Autodesk Inventor part; units mm, degrees
ref_plane "XZ Plane" through (0, 0, 0) normal (0, 1, 0) x (-1, 0, 0)
ref_plane "XY Plane" through (0, 0, 0) normal (0, 0, 1) x (1, 0, 0)
sketch "Sketch1" plane through (0, 0, 0) normal (0, 1, 0) x (-1, 0, 0)
  line L0 (0, 0) -> (0, -405.743) construction
  line L1 (-4, 0) -> (-4, -405.743)
  line L2 (4, -405.743) -> (4, 0)
  arc A0 (4, 0) -> (-4, 0) centre (0, 0) ccw
  arc A1 (-4, -405.743) -> (4, -405.743) centre (0, -405.743) ccw
  circle A2 centre (0, 0) radius 1.5
  circle A3 centre (0, -405.743) radius 1.5
  line L3 (0, -347.063) -> (0, -288.743) construction
  line L4 (1.5, -347.063) -> (1.5, -288.743)
  line L5 (-1.5, -288.743) -> (-1.5, -347.063)
  arc A4 (-1.5, -347.063) -> (1.5, -347.063) centre (0, -347.063) ccw
  arc A5 (1.5, -288.743) -> (-1.5, -288.743) centre (0, -288.743) ccw
  line L6 (0, -405.743) -> (0, -505.743) construction
  line L7 (-4, -405.743) -> (-4, -505.743)
  line L8 (4, -505.743) -> (4, -405.743)
  arc A6 (4, -405.743) -> (-4, -405.743) centre (0, -405.743) ccw
  arc A7 (-4, -505.743) -> (4, -505.743) centre (0, -505.743) ccw
  point P0 (0, -202.8715)
  point P1 (0, -317.903)
  point P2 (0, -455.743)
  dimension "d0" = 8
  dimension "d1" = 405.743
  dimension "d2" = 3
  dimension "d3" = 3
  dimension "d20" = 3
  dimension "d21" = 58.68
  dimension "d22" = 117
  dimension "d23" = 8
  dimension "d24" = 100
extrude "Extrusion1" add sketch "Sketch1" along normal blind 6
sketch "Sketch2" plane through (0, 6, 0) normal (0, 1, 0) x (1, 0, 0)
  line L0 (-4, 505.743) -> (-4, 0)
  arc A0 (-4, 0) -> (4, 0) centre (0, 0) ccw
  line L1 (4, 0) -> (4, 505.743)
  arc A1 (4, 505.743) -> (-4, 505.743) centre (0, 505.743) ccw
  arc A2 (1.5, 347.063) -> (-1.5, 347.063) centre (0, 347.063) ccw
  line L2 (1.5, 347.063) -> (1.5, 288.743)
  arc A3 (-1.5, 288.743) -> (1.5, 288.743) centre (0, 288.743) ccw
  line L3 (-1.5, 288.743) -> (-1.5, 347.063)
  circle A4 centre (0, 405.743) radius 1.5
  circle A5 centre (0, 0) radius 1.5
  line L4 (-4, 505.743) -> (-4, 0)
  line L5 (-4, 252.8715) -> (0, 244.2935)
  line L6 (0, 244.2935) -> (4, 252.8715)
  line L7 (4, 0) -> (4, 505.743)
  dimension "d25" = 25
  dimension "d26" = 25
extrude "Extrusion2" [suppressed]
CAD build for the part. Positions are in the model's coordinates, mm. Coordinates: 2 decimals unless noted, no trailing zeros. Order: outer loops, then holes, each group sorted by start corner. A loop starts at its lowest first (then second) coordinate and runs counter-clockwise, first axis right, second up.
(1) Saw through at B-B, the plane y = 2.4. Write the cut outline in (x, z), and give its area (3 significant figures).
Solution:
outline: (-4, -505.74) arc R4 ccw to (4, -505.74) - (4, 0) arc R4 ccw to (-4, 0) - close; hole circle Ø3 at (0, -405.74); hole (-1.5, -347.06) arc R1.5 ccw to (1.5, -347.06) - (1.5, -288.74) arc R1.5 ccw to (-1.5, -288.74) - close; hole circle Ø3 at (0, 0)
area: 3,900 mm2
(2) Pin check, flat tip, straight feed: pin 1 Ø1.5 at (x, y) = (3, 3) entering from -Z. Stop position of the tip, or through.
Solution:
pin 1: stops at z = -509.05
(3) Drill centre lines: L1, parallel to Z at x = 0, y = 4.3; L2, parallel to Z at x = -1.25, y = 3.4; L3, parallel to X at y = 3.1, z = -340.5. Where is each one in solid material? Low to high.
Solution:
L1: z = -509.74 to -407.24, -404.24 to -348.56, -287.24 to -1.5, 1.5 to 4
L2: z = -509.54 to -406.57, -404.91 to -347.89, -287.91 to -0.83, 0.83 to 3.8
L3: x = -4 to -1.5, 1.5 to 4
(4) Saw through at A-A, the plane x = 0. Write the cut outline in (y, z), and give its area (3 significant figures).
Solution:
outline: (0, -509.74) - (6, -509.74) - (6, -407.24) - (0, -407.24) - close; (0, -404.24) - (6, -404.24) - (6, -348.56) - (0, -348.56) - close; (0, -287.24) - (6, -287.24) - (6, -1.5) - (0, -1.5) - close; (0, 1.5) - (6, 1.5) - (6, 4) - (0, 4) - close
area: 2,680 mm2
(5) Mould opens along Y. For faces 1 (the face through (0, 6, -249)), 2 (the face through (0, 0, -249)) say: released by +Y, released by -Y, zero draft, split by the parting line, or undercut.
Solution:
face 1: released by +Y
face 2: released by -Y
